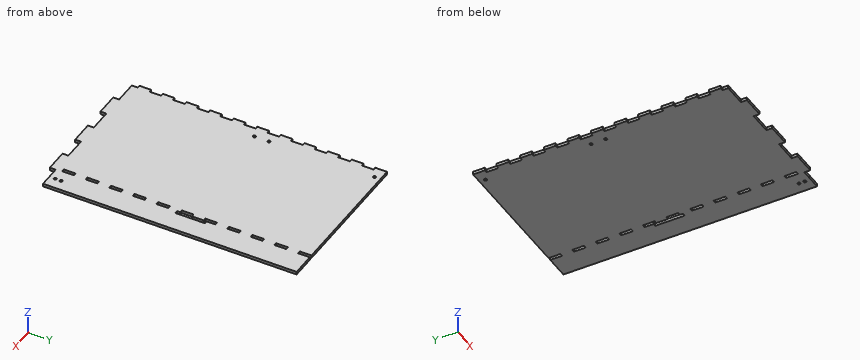
```python
from build123d import *

# Parameters (mm, degrees)
SKETCH1_W           = 3.175
SKETCH1_H           = 12.734636364
SKETCH1_H_2         = 12.734636363
BOSS_EXTRUDE1_DEPTH = 3.175
SKETCH2_R           = 1.5
SKETCH2_W           = 3.175
SKETCH2_H           = 31.877
CUT_EXTRUDE1_DEPTH  = 4.175


with BuildPart() as part:
    # Sketch1 → Boss-Extrude1 (new body)
    with BuildSketch(Plane.XY):
        Polygon((24.429357143, -133.731), (24.429357143, -140.081), (48.858714286, -140.081), (48.858714286, -133.731), (73.288071429, -133.731), (73.288071429, -140.081), (97.717428571, -140.081), (97.717428571, -133.731), (122.146785714, -133.731), (122.146785714, -140.081), (146.576142857, -140.081), (146.576142857, -133.731), (171.0055, -133.731), (171.0055, 140.081), (145.6055, 140.081), (145.6055, 127.346363636), (142.4305, 127.346363636), (142.4305, 140.081), (-3.175, 140.081), (-3.175, 127.346363636), (0, 127.346363636), (0, 114.611727273), (-3.175, 114.611727273), (-3.175, 101.877090909), (0, 101.877090909), (0, 89.142454545), (-3.175, 89.142454545), (-3.175, 76.407818182), (0, 76.407818182), (0, 63.673181818), (-3.175, 63.673181818), (-3.175, 50.938545455), (0, 50.938545455), (0, 38.203909091), (-3.175, 38.203909091), (-3.175, 25.469272727), (0, 25.469272727), (0, 12.734636364), (-3.175, 12.734636364), (-3.175, 0), (0, 0), (0, -12.734636364), (-3.175, -12.734636364), (-3.175, -25.469272727), (0, -25.469272727), (0, -38.203909091), (-3.175, -38.203909091), (-3.175, -50.938545455), (0, -50.938545455), (0, -63.673181818), (-3.175, -63.673181818), (-3.175, -76.407818182), (0, -76.407818182), (0, -89.142454545), (-3.175, -89.142454545), (-3.175, -101.877090909), (0, -101.877090909), (0, -114.611727273), (-3.175, -114.611727273), (-3.175, -127.346363636), (0, -127.346363636), (0, -133.731), align=None)
        with Locations((144.018, 108.244409091)):
            Rectangle(SKETCH1_W, SKETCH1_H, mode=Mode.SUBTRACT)
        with Locations((144.018, -120.979045455)):
            Rectangle(SKETCH1_W, SKETCH1_H_2, mode=Mode.SUBTRACT)
        with Locations((144.018, -95.509772727)):
            Rectangle(SKETCH1_W, SKETCH1_H, mode=Mode.SUBTRACT)
        with Locations((144.018, -70.0405)):
            Rectangle(SKETCH1_W, SKETCH1_H, mode=Mode.SUBTRACT)
        with Locations((144.018, -44.571227273)):
            Rectangle(SKETCH1_W, SKETCH1_H, mode=Mode.SUBTRACT)
        with Locations((144.018, -19.101954545)):
            Rectangle(SKETCH1_W, SKETCH1_H_2, mode=Mode.SUBTRACT)
        with Locations((144.018, 6.367318182)):
            Rectangle(SKETCH1_W, SKETCH1_H, mode=Mode.SUBTRACT)
        with Locations((144.018, 31.836590909)):
            Rectangle(SKETCH1_W, SKETCH1_H, mode=Mode.SUBTRACT)
        with Locations((144.018, 57.305863637)):
            Rectangle(SKETCH1_W, SKETCH1_H_2, mode=Mode.SUBTRACT)
        with Locations((144.018, 82.775136363)):
            Rectangle(SKETCH1_W, SKETCH1_H_2, mode=Mode.SUBTRACT)
    extrude(amount=BOSS_EXTRUDE1_DEPTH)

    # Sketch2 → Cut-Extrude1 (cut, through all)
    with BuildSketch(Plane.XY.offset(3.175)):
        with Locations((158.790821429, -121.031)):
            Circle(SKETCH2_R)
        with Locations((11.1125, 20.574)):
            Circle(SKETCH2_R)
        with Locations((11.1125, 4.826)):
            Circle(SKETCH2_R)
        with Locations((158.790821429, -127.381)):
            Circle(SKETCH2_R)
        with Locations((9.525, 133.731)):
            Circle(SKETCH2_R)
        with Locations((147.193, 12.7)):
            Rectangle(SKETCH2_W, SKETCH2_H)
    extrude(amount=-CUT_EXTRUDE1_DEPTH, mode=Mode.SUBTRACT)


solid = part.part
```
Geometry: final body of the model. Coordinates: model frame, mm. Coordinates: 2 decimals unless noted, no trailing zeros. Loops run counter-clockwise (first coordinate to the right, second up) from the corner with the lowest first, then second, coordinate; pieces in that order, holes last. Notation, with made-up numbers: (-11.5, -15.75) -> (8.5, -15.75) arc R13 cw to (8.5, 7.25) -> close; hole circle Ø8 at (77.25, 54.5). An arc over 180 degrees is marked (long way). Use a Markdown table: item, result. Add a question column.
(1) Section query D-D, the plane z = 1.25. State how many separate pieces and enclosed holes the cut face has, plus the area to 3 significant figures.
(2) Section query B-B, the plane x = 68. Return loops of the section in (y, z) (3 decimals), plus the area to 3 significant figures.
(3) Pin query (flat end, axial travel): pin 1 Ø1.6 at (x, z) = (159.5, 2) entering from -Y; pin 2 Ø1.6 at (x, z) = (-1.5, 1.5) entering from -Y; pin 3 Ø1.6 at (y, z) = (-137.5, 1) entering from -X. Return the tip coordinate at first contact, or that it passes through.
(4) Section query A-A, the plane y = 80. Return loops of the section in (x, z) (1 decimal).
(5) Line query: line 1 along X through (y, z) = (20.5, 1.75); line 2 along X through (y, z) = (108.5, 2.6) (1 decimal); line 3 along X through (y, z) = (14, 1.9). Output: solid intervals per line, ascending.
(6) Section query C-C, the plane y = -59. Return loops of the section in (x, z) (1 decimal), plus the area to 3 significant figures.
Answer:
| question | item | result |
|---|---|---|
| 1 | separate pieces | 1 |
| 1 | enclosed holes | 14 |
| 1 | area | 47,200 mm^2 |
| 2 | outline | (-133.731, 0) -> (140.081, 0) -> (140.081, 3.175) -> (-133.731, 3.175) -> close |
| 2 | area | 869 mm^2 |
| 3 | pin 1 | stops at y = -133.73 |
| 3 | pin 2 | stops at y = -127.35 |
| 3 | pin 3 | stops at x = 24.43 |
| 4 | outline | (-3.2, 0) -> (142.4, 0) -> (142.4, 3.2) -> (-3.2, 3.2) -> close; (145.6, 0) -> (171, 0) -> (171, 3.2) -> (145.6, 3.2) -> close |
| 5 | line 1 | x = 0 to 9.61, 12.61 to 145.61, 148.78 to 171.01 |
| 5 | line 2 | x = -3.2 to 142.4, 145.6 to 171 |
| 5 | line 3 | x = 0 to 145.61, 148.78 to 171.01 |
| 6 | outline | (0, 0) -> (171, 0) -> (171, 3.2) -> (0, 3.2) -> close |
| 6 | area | 543 mm^2 |
